Autodesk Inventor part; units mm, degrees
ref_plane "YZ Plane" through (0, 0, 0) normal (1, 0, 0) x (0, 1, 0)
ref_plane "XZ Plane" through (0, 0, 0) normal (0, 1, 0) x (-1, 0, 0)
ref_plane "XY Plane" through (0, 0, 0) normal (0, 0, 1) x (1, 0, 0)
sketch "Sketch1" plane through (0, 0, 0) normal (0, 0, 1) x (1, 0, 0)
  circle A0 centre (0, 0) radius 7.5
  dimension "d0" = 15
extrude "Extrusion1" add sketch "Sketch1" along normal mid plane 250
sketch "Sketch2" plane through (0, 0, 125) normal (0, 0, 1) x (1, 0, 0)
  circle A0 centre (0, 0) radius 7.5
  circle A1 centre (0, 0) radius 11
  dimension "d3" = 22
extrude "Extrusion2" add sketch "Sketch2" along normal blind 14 contours A0 | A1
fillet "Fillet1" radius 2 2 edges at (-11, 0, 125) (-7.5, 0, 125)
fillet "Fillet2" radius 4 1 edges at (-11, 0, 139)
chamfer "Chamfer1" distance 2 angle 45 1 edges at (-7.5, 0, -125)
thread "Thread1"
properties part number "HANDLE" material "Steel, Mild"
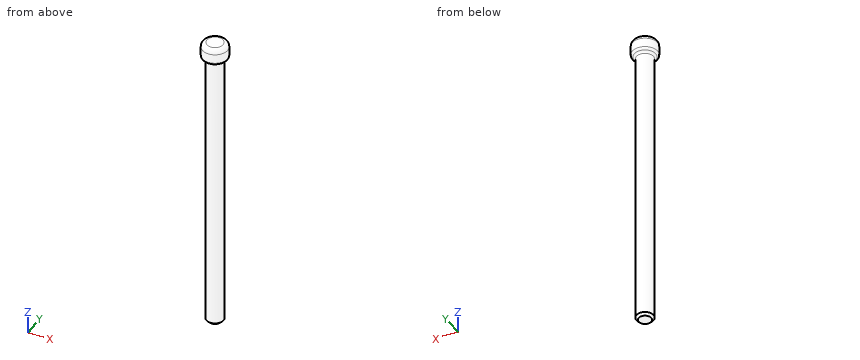
Could you check a few things on this model? Use its own coordinates, in mm. Coordinates: 2 decimals unless noted, no trailing zeros. Write each loop counter-clockwise with the first axis right and the second up, starting at its lowest first coordinate (ties: lowest second). Pieces come first, ordered by that corner, then holes. Notation, with made-up numbers: (47.5, 80) - (96.5, 80) arc R16 cw to (96.5, 90) - close; hole circle Ø4 at (-6, 38.5). An arc over 180 degrees is marked (long way). Put each result on its own line as item: value. Start each with the question number.
Q1. I'm going to push flat-ended pins straight in: P1, Ø6, axis at y = 2.5, z = 53.5, coming from the +X side; P2, Ø3, axis at x = -8.5, y = 8.5, coming from the -Z side; P3, Ø1.5, axis at y = -5.5, z = 49, coming from the -X side. Where does each tip first touch, or does it pass through?
Q2. Please list where these lines run through material, in increasing order: L1, parallel to Y at x = 0.75, z = 116.5; L2, parallel to Z at x = 1.25, y = 6.75; L3, parallel to Y at x = -6.75, z = 113.5.
Q3. I want a section at A-A on z = -99.5. Write out the boundary of the cut face in (x, y), plus the area to 3 significant figures.
Checks:
1. P1: x = 7.5
1. P2: z = 125.7
1. P3: x = -5.8
2. L1: -7.46 to 7.46
2. L2: -123.64 to 139
2. L3: -3.27 to 3.27
3. outline: circle Ø15 at (0, 0)
3. area: 177 mm²
